```python
from build123d import *

# Parameters (mm, degrees)
CROQUIS1_W              = 400
CROQUIS1_H              = 400
CROQUIS1_R              = 3
SALIENTE_EXTRUIR1_DEPTH = 5
CHAFL_N1_SIZE           = 2
CORTAR_EXTRUIR1_DEPTH   = 10


with BuildPart() as part:
    # Croquis1 → Saliente-Extruir1 (new body)
    with BuildSketch(Plane(origin=(0, 0, 0), x_dir=(1, 0, 0), z_dir=(0, 1, 0))):
        with Locations((11.673151751, -29.571984436)):
            Rectangle(CROQUIS1_W, CROQUIS1_H)
        with Locations(Location((-173.326848249, 120.428015564, 0), (0, 0, 270))):
            Circle(CROQUIS1_R, mode=Mode.SUBTRACT)
        with Locations(Location((-173.326848249, -199.571984436, 0), (0, 0, 270))):
            Circle(CROQUIS1_R, mode=Mode.SUBTRACT)
        with Locations(Location((196.673151751, -199.571984436, 0), (0, 0, 270))):
            Circle(CROQUIS1_R, mode=Mode.SUBTRACT)
        with Locations(Location((196.673151751, 120.428015564, 0), (0, 0, 270))):
            Circle(CROQUIS1_R, mode=Mode.SUBTRACT)
        with Locations(Location((-173.326848249, -39.571984436, 0), (0, 0, 270))):
            Circle(CROQUIS1_R, mode=Mode.SUBTRACT)
        with Locations(Location((196.673151751, -39.571984436, 0), (0, 0, 270))):
            Circle(CROQUIS1_R, mode=Mode.SUBTRACT)
        with Locations(Location((-88.326848249, 155.428015564, 0), (0, 0, 270))):
            Circle(CROQUIS1_R, mode=Mode.SUBTRACT)
        with Locations(Location((111.673151751, 155.428015564, 0), (0, 0, 270))):
            Circle(CROQUIS1_R, mode=Mode.SUBTRACT)
    extrude(amount=SALIENTE_EXTRUIR1_DEPTH)

    # Chaflán1
    chafl_n1_edges = [part.edges().sort_by_distance(p)[0] for p in [
        (11.673151751, 0, -170.428015564),
        (211.673151751, 0, 29.571984436),
        (11.673151751, 0, 229.571984436),
        (-188.326848249, 0, 29.571984436),
    ]]
    chamfer(chafl_n1_edges, length=CHAFL_N1_SIZE)

    # Croquis2 → Cortar-Extruir1 (cut)
    with BuildSketch(Plane(origin=(0, 5, 0), x_dir=(1, 0, 0), z_dir=(0, 1, 0))):
        Polygon((-91.777504567, 17.93962644), (-133.486350664, -34.097124404), (-121.499339941, 41.762471587), align=None)
        Polygon((-120.940367697, 45.29991804), (-66.966286679, 67.345973172), (52.354078092, 10.388168385), (-17.091461921, -39.85772233), align=None)
        Polygon((163.775185266, -73.593412395), (52.354078092, 6.009139456), (-13.604376997, -41.724802745), (89.090925469, -62.956955386), align=None)
        Polygon((31.311804468, -55.660536224), (10.169460209, -128.358580052), (-13.558867473, -114.834434958), (-11.835173214, -45.882080038), align=None)
        Polygon((7.646392173, -130.362582514), (-49.989323249, -137.40209781), (-15.003820451, -117.452917491), align=None)
        Polygon((-94.005890503, 11.316220426), (-21.421222894, -49.654322149), (-23.868784692, -109.619586204), (-16.697922209, -113.650656174), (-15.003820451, -45.882080038), (-19.79537186, -43.31560542), (-89.832558674, 16.28451972), align=None)
        Polygon((-25.572304789, -111.697520158), (-51.931593577, -128.358580052), (-37.17095608, -126.84931671), (-18.323489891, -115.772410748), align=None)
    extrude(amount=-CORTAR_EXTRUIR1_DEPTH, mode=Mode.SUBTRACT)


solid = part.part
```
Model file for the job. Use its own axes, mm. A direction names the side the tool comes from. Coordinates: 2 decimals unless noted, no trailing zeros. Order: outer loops, then holes, each group sorted by start corner. A loop starts at its lowest first (then second) coordinate and runs counter-clockwise, first axis right, second up. Notation, with made-up numbers: M 39.5,85.25 L 79.5,85.25 A17 ccw 79.5,101.25 Z; hole C 68.5,-40 d11. An arc over 180 degrees is marked long. Answer as CSV lines item,"result".
(1) Flat gauge pin, fed straight in: pin 1 (5 mm diameter, centred on x = 196.67, z = -120.43, fed in from +Y). Where does the tip first touch, or does it go through?
Geometry says:
pin 1,"passes through"
(2) Band-saw the part on B-B, the plane x = 102.5. List the corners of the cut face in (y, z).
Geometry says:
outline,"M 0,-168.43 L 2,-170.43 L 5,-170.43 L 5,29.82 L 0,29.82 Z; M 0,64.87 L 5,64.87 L 5,229.57 L 2,229.57 L 0,227.57 Z"
(3) Band-saw the part on A-A, the plane x = -79. List the corners of the cut face in (y, z).
Geometry says:
outline,"M 0,-168.43 L 2,-170.43 L 5,-170.43 L 5,-62.43 L 0,-62.43 Z; M 0,-10.91 L 5,-10.91 L 5,-7.07 L 0,-7.07 Z; M 0,1.29 L 5,1.29 L 5,229.57 L 2,229.57 L 0,227.57 Z"
(4) Wall check: line 1 along X through (y, z) = (0.65, 79); line 2 along Z through (x, y) = (-112, 0.9); line 3 along X through (y, z) = (4.1, 39). Give the ranges that are in metal, low to high.
Geometry says:
line 1,"x = -186.98 to -22.62, -15.83 to -12.66, 24.52 to 210.32"
line 2,"z = -169.33 to -48.95, -37.97 to -34.15, 7.29 to 228.47"
line 3,"x = -188.33 to -176.27, -170.38 to -34.11, -24.87 to -18.14, -15.91 to -9.84, 115.35 to 193.73, 199.62 to 211.67"
(5) Pull direction X, two halves, no side cores. Call faces 1 (the flat face through (-3.837, 2.535, 123.817)), 2 (the flat face through (-35, 0, 27)): +X half, -X half, draft (parallel to the pull), parting line (faces both ways), or undercut.
Geometry says:
face 1,"undercut"
face 2,"draft"
(6) Band-saw the part on D-D, the plane y = 3.8. State how many separate pieces and enclosed holes the cut face has, then the cut area to 3 significant figures.
Geometry says:
separate pieces,"1"
enclosed holes,"15"
area,"140,000 mm2"
(7) 3-axis set-ups, long thin cutter, end or side, ignore diameter. For faces 3 (the flat face through (108.845, 2.535, 34.349)), 4 (the flat face through (-36, 5, 27)): which of +Z, -Z, +X, -X, +Y, -Y reach the whole face in a straight line?
Geometry says:
face 3,"+Y, -Y"
face 4,"+Z, -Z, +X, -X, +Y"
(8) Band-saw the part on C-C, the plane x = 144. List the corners of the cut face in (y, z), then the cut area to 3 significant figures.
Geometry says:
outline,"M 0,-168.43 L 2,-170.43 L 5,-170.43 L 5,59.47 L 0,59.47 Z; M 0,70.78 L 5,70.78 L 5,229.57 L 2,229.57 L 0,227.57 Z"
area,"1,940 mm2"
